CAD build for the part. Positions are in the model's coordinates, mm. A direction names the side the tool comes from. Coordinates: 2 decimals unless noted, no trailing zeros. Loops run counter-clockwise (first coordinate to the right, second up) from the corner with the lowest first, then second, coordinate; pieces in that order, holes last. Notation, with made-up numbers: (4, -16) -> (47, -16) arc R25 ccw to (47, 12) -> close; hole circle Ø11 at (50, -3). An arc over 180 degrees is marked (long way). Return JSON: item names as keys, results as strings. Group by question number.
(1) Saw through at D-D on z = 14.75. Write the cut outline in (x, y), then the cut area to 3 significant figures.
(2) Saw through at B-B on x = 148. Write the cut outline in (y, z).
(3) Mould opens along Z. For faces 1 (the face through (146, -37, 10)), 2 (the face through (64, 32, 20)), 3 (the face through (-17, -36, 10)) say: pulls with the +Z half, pulls with the -Z half, needs draft (parallel to the pull), parting line crosses it, or undercut.
(4) Probe L1, parallel to Z at x = 148, y = 33; L2, parallel to Y at x = 77, z = 11.5; L3, parallel to X at y = 15.5, z = 10. List the from-to ranges inside material, lowest first.
(5) Saw through at A-A on x = 42.5. Write the cut outline in (y, z), then the cut area to 3 significant figures.
(6) Flat gauge pins, fed straight in: pin 1 Ø6.5 at (x, z) = (-5, 10) entering from +Y; pin 2 Ø7.5 at (x, z) = (-14, 7) entering from -Y; pin 3 Ø12 at (y, z) = (5, 13) entering from +X; pin 4 Ø2 at (y, z) = (-41, 14.5) entering from -X. Where does each tip first touch, or does it go through?
(7) Saw through at C-C on y = -16. Write the cut outline in (x, z).
(8) Tool access for faces 4 (the face through (0, -0.4, 7.6)), 5 (the face through (-13, 38.5, 10)), 6 (the face through (-10, 0.5, 12.1)): list every direction of +Z, -Z, +X, -X, +Y, -Y with a clear straight run to the whole face (end or side of a thin tool).
```python
from build123d import *

# Parameters (mm, degrees)
PAD_DEPTH       = 20
SKETCH004_R     = 2
POCKET002_DEPTH = 168.001
SKETCH005_R     = 2
POCKET003_DEPTH = 85.001


with BuildPart() as part:
    # Sketch → Pad (new body)
    with BuildSketch(Plane.XY):
        Polygon((-10, -42.5), (158, -42.5), (158, -30.5), (0, -30.5), (0, 30.5), (158, 30.5), (158, 42.5), (-10, 42.5), (-10, 38.5), (-17, 38.5), (-17, 33.5), (-10, 33.5), (-10, -33.5), (-17, -33.5), (-17, -38.5), (-10, -38.5), align=None)
    extrude(amount=PAD_DEPTH)

    # Sketch004 → Pocket002 (cut, through all)
    with BuildSketch(Plane(origin=(-10, 0, 0), x_dir=(0, -1, 0), z_dir=(-1, 0, 0))):
        with Locations((0, 10)):
            Circle(SKETCH004_R)
    extrude(amount=-POCKET002_DEPTH, mode=Mode.SUBTRACT)

    # Sketch005 → Pocket003 (cut, through all)
    with BuildSketch(Plane.XZ.offset(42.5)):
        with Locations((-5, 10)):
            Circle(SKETCH005_R)
        with Locations((148, 10)):
            Circle(SKETCH005_R)
    extrude(amount=-POCKET003_DEPTH, mode=Mode.SUBTRACT)


solid = part.part
```
Geometry results:
{
 "1": {"outline": "(-17, -38.5) -> (-10, -38.5) -> (-10, -42.5) -> (158, -42.5) -> (158, -30.5) -> (0, -30.5) -> (0, 30.5) -> (158, 30.5) -> (158, 42.5) -> (-10, 42.5) -> (-10, 38.5) -> (-17, 38.5) -> (-17, 33.5) -> (-10, 33.5) -> (-10, -33.5) -> (-17, -33.5) -> close", "area": "4,710 mm²"},
 "2": {"outline": "(-42.5, 0) -> (-30.5, 0) -> (-30.5, 8) -> (-42.5, 8) -> close; (-42.5, 12) -> (-30.5, 12) -> (-30.5, 20) -> (-42.5, 20) -> close; (30.5, 0) -> (42.5, 0) -> (42.5, 8) -> (30.5, 8) -> close; (30.5, 12) -> (42.5, 12) -> (42.5, 20) -> (30.5, 20) -> close"},
 "3": {"face 1": "undercut", "face 2": "pulls with the +Z half", "face 3": "needs draft"},
 "4": {"L1": "0 to 8, 12 to 20", "L2": "-42.5 to -30.5, 30.5 to 42.5", "L3": "-10 to -7, -3 to 0"},
 "5": {"outline": "(-42.5, 0) -> (-30.5, 0) -> (-30.5, 20) -> (-42.5, 20) -> close; (30.5, 0) -> (42.5, 0) -> (42.5, 20) -> (30.5, 20) -> close", "area": "480 mm²"},
 "6": {"pin 1": "y = 42.5", "pin 2": "y = -38.5", "pin 3": "x = 0", "pin 4": "x = -10"},
 "7": {"outline": "(-10, 0) -> (0, 0) -> (0, 20) -> (-10, 20) -> close; hole circle Ø4 at (-5, 10)"},
 "8": {"face 4": "+Z, -Z, +X", "face 5": "+Z, -Z, -X, +Y", "face 6": "+Z, -Z, -X"}
}
